CAD build for the part. Positions are in the model's coordinates, mm. A direction names the side the tool comes from. Round coordinates to 2 decimals unless told otherwise and drop trailing zeros. Loops run counter-clockwise (first coordinate to the right, second up) from the corner with the lowest first, then second, coordinate; pieces in that order, holes last.
```python
from build123d import *
from build123d import SkipClean  # not in build123d's __all__

# Parameters (mm, degrees)
F0_R     = 19.05
F0_R_2   = 2.15265
F1_DEPTH = 66.04
F3_DEPTH = 66.04
F4_COUNT = 4
F4_ANGLE = 270
F5_R     = 2.15265
F5_R_2   = 7.9375
F6_DEPTH = 7.9375
F8_DEPTH = 25.4


# Not quite as in the source:
# - after a boolean that leaves OpenCascade's solid faulty, fix() repairs it


with BuildPart() as f1:
    # F0 (on Top) → F1 (new body)
    with BuildSketch(Plane.XY):
        Circle(F0_R)
        with Locations((-9.5415221286, -9.5415221286)):
            Circle(F0_R_2, mode=Mode.SUBTRACT)
        with Locations((9.5415221286, -9.5415221286)):
            Circle(F0_R_2, mode=Mode.SUBTRACT)
        with Locations((-9.5415221286, 9.5415221286)):
            Circle(F0_R_2, mode=Mode.SUBTRACT)
        with BuildLine():
            ThreePointArc((0, 7.9375), (5.6126600757, 5.6126600757), (7.9375, 0))
            ThreePointArc((7.9375, 0), (-5.6126600757, -5.6126600757), (0, 7.9375))
        make_face(mode=Mode.SUBTRACT)
        with Locations((9.5415221286, 9.5415221286)):
            Circle(F0_R_2, mode=Mode.SUBTRACT)
    extrude(amount=F1_DEPTH)

    # F2 (on face) → F3 (cut, through all)
    with BuildSketch(Plane(origin=(0, 0, 0), x_dir=(1, 0, 0), z_dir=(0, 0, -1))):
        with BuildLine():
            ThreePointArc((8.8488960712, -15.0544327217), (5.6543471209, -13.5116335278), (4.0444600337, -10.350362278))
            ThreePointArc((4.0444600337, -10.350362278), (0, -11.1125), (-4.0444600337, -10.350362278))
            ThreePointArc((-4.0444600337, -10.350362278), (-5.6543471209, -13.5116335278), (-8.8488960712, -15.0544327217))
            ThreePointArc((-8.8488960712, -15.0544327217), (0, -17.4625), (8.8488960712, -15.0544327217))
        make_face()
    f3 = extrude(amount=-F3_DEPTH, mode=Mode.SUBTRACT)

    # F4: F3 ×4 about axis
    f4_axis = Axis((0, 0, 0), (0, 0, -1))
    for i in range(1, F4_COUNT):
        add(f3.rotate(f4_axis, i * F4_ANGLE / (F4_COUNT - 1)), clean=False, mode=Mode.SUBTRACT)

    # F5 (on face) → F6 (join)
    with BuildSketch(Plane.XY.offset(66.04)):
        with BuildLine():
            Line((35.4737477046, -58.7862808051), (18.4008869908, 4.9305028092))
            ThreePointArc((18.4008869908, 4.9305028092), (13.4703841816, 13.4703841816), (4.9305028092, 18.4008869908))
            Line((4.9305028092, 18.4008869908), (-58.7862808051, 35.4737477046))
            ThreePointArc((-58.7862808051, 35.4737477046), (-61.9475900585, 35.228016284), (-64.2539485249, 33.05201749))
            ThreePointArc((-64.2539485249, 33.05201749), (-51.093080555, -51.093080555), (33.05201749, -64.2539485249))
            ThreePointArc((33.05201749, -64.2539485249), (35.228016284, -61.9475900585), (35.4737477046, -58.7862808051))
        make_face()
        with Locations((-9.5415221286, -9.5415221286)):
            Circle(F5_R, mode=Mode.SUBTRACT)
        Circle(F5_R_2, mode=Mode.SUBTRACT)
        with Locations((9.5415221286, -9.5415221286)):
            Circle(F5_R, mode=Mode.SUBTRACT)
        with Locations((-9.5415221286, 9.5415221286)):
            Circle(F5_R, mode=Mode.SUBTRACT)
        with Locations((9.5415221286, 9.5415221286)):
            Circle(F5_R, mode=Mode.SUBTRACT)
    with SkipClean():  # cleaning this boolean's faces spoils the solid; the shape is the same uncleaned
        extrude(amount=F6_DEPTH)

    # F7 (on face) → F8 (join)
    with BuildSketch(Plane.XY.offset(73.9775)):
        with BuildLine():
            ThreePointArc((-55.7838644899, 28.6950344237), (-57.8404149742, 35.1085679744), (-64.2539485249, 33.05201749))
            ThreePointArc((-64.2539485249, 33.05201749), (-51.093080555, -51.093080555), (33.05201749, -64.2539485249))
            ThreePointArc((33.05201749, -64.2539485249), (35.1085679744, -57.8404149742), (28.6950344237, -55.7838644899))
            ThreePointArc((28.6950344237, -55.7838644899), (-44.3578884642, -44.3578884642), (-55.7838644899, 28.6950344237))
        make_face()
    extrude(amount=F8_DEPTH)

    add(f1.part.fix(), mode=Mode.REPLACE)


solid = f1.part
```
Item 1: Cut at C-C, the plane y = -21.5. Give the cut face in (x, z).
Answers follow:
outline: (-68.98, 66.04) - (25.48, 66.04) - (25.48, 73.98) - (-58.93, 73.98) - (-58.93, 99.38) - (-68.98, 99.38) - close
Item 2: Flat gauge pins, fed straight in: P1, Ø1.5, axis at y = -43, z = 72, coming from the +X side; P2, Ø7, axis at x = -9.54, y = -9.54, coming from the +Z side; P3, Ø8, axis at y = -8.5, z = 40.5, coming from the +X side. Where does each tip first touch, or does it go through?
Answers follow:
P1: stops at x = 31.44
P2: stops at z = 73.98
P3: stops at x = 18.51
Item 3: Probe line 1 (X direction, y = 1, z = 85); line 2 (Z direction, x = -32.5, y = -10); line 3 (Y direction, x = -12.5, z = 13). List the from-to ranges inside material, lowest first.
Answers follow:
line 1: x = -72.25 to -62.72
line 2: z = 66.04 to 73.98
line 3: y = -14.38 to -4.84, 4.84 to 14.38
Item 4: Cut at A-A, the plane z = 47.5. State how many separate pieces and enclosed holes the cut face has, plus the area to 3 significant figures.
Answers follow:
separate pieces: 1
enclosed holes: 9
area: 584 mm2
Item 5: Cut at D-D, the plane x = -33. Give the cut face in (y, z), plus the area to 3 significant figures.
Answers follow:
outline: (-64.28, 66.04) - (28.56, 66.04) - (28.56, 73.98) - (-53.35, 73.98) - (-53.35, 99.38) - (-64.28, 99.38) - close
area: 1,010 mm2
Item 6: Cut at B-B, the plane y = -2. Give the cut face in (x, z).
Answers follow:
outline: (-72.23, 66.04) - (-18.94, 66.04) - (-18.94, 0) - (-17.35, 0) - (-17.35, 66.04) - (-10.93, 66.04) - (-10.93, 0) - (-7.68, 0) - (-7.68, 73.98) - (-62.7, 73.98) - (-62.7, 99.38) - (-72.23, 99.38) - close; (7.68, 0) - (10.93, 0) - (10.93, 66.04) - (17.35, 66.04) - (17.35, 0) - (18.94, 0) - (18.94, 66.04) - (20.26, 66.04) - (20.26, 73.98) - (7.68, 73.98) - close
Item 7: 3-axis set-ups, long thin cutter, end or side, ignore diameter. For faces 1 (the cylindrical face through (-51.99, -50.18, 82.48)), 2 (the cylindrical face through (10.241, 16.063, 36.471)): which of +Z, -Z, +X, -X, +Y, -Y reach the whole face in a straight line?
Answers follow:
face 1: +Z, -Z
face 2: -Z
Item 8: Two-plate mould, pull along X, no slides. Class faces 3 (the cylindrical face through (11.112, -0.058, 32.558)), 4 (the flat face through (-26.482, 26.818, 69.953)), 5 (the flat face through (8.2, 0.3, 0)): released by +X, released by -X, zero draft, split by the parting line, or undercut.
Answers follow:
face 3: undercut
face 4: released by +X
face 5: zero draft
